Autodesk Inventor part; units mm, degrees
ref_plane "YZ Plane" through (0, 0, 0) normal (1, 0, 0) x (0, 1, 0)
ref_plane "XZ Plane" through (0, 0, 0) normal (0, 1, 0) x (-1, 0, 0)
ref_plane "XY Plane" through (0, 0, 0) normal (0, 0, 1) x (1, 0, 0)
sketch "Sketch1" plane through (0, 0, 0) normal (0, 0, 1) x (1, 0, 0)
  line L0 (0, 0) -> (101.4, 0)
  line L1 (101.4, 0) -> (101.4, 50)
  line L2 (101.4, 50) -> (0, 50)
  line L3 (0, 50) -> (0, 0)
  circle A0 centre (50.7, 25) radius 3.75
  line L4 (2.5, 36.45) -> (2.5, 13.55) construction
  line L5 (1.45, 36.45) -> (1.45, 13.55)
  line L6 (3.55, 13.55) -> (3.55, 36.45)
  arc A1 (3.55, 36.45) -> (1.45, 36.45) centre (2.5, 36.45) ccw
  arc A2 (1.45, 13.55) -> (3.55, 13.55) centre (2.5, 13.55) ccw
  line L7 (101.4, 50) -> (101.4, 0)
  line L8 (98.9, 36.45) -> (98.9, 13.55) construction
  line L9 (99.95, 36.45) -> (99.95, 13.55)
  line L10 (97.85, 13.55) -> (97.85, 36.45)
  arc A3 (99.95, 36.45) -> (97.85, 36.45) centre (98.9, 36.45) ccw
  arc A4 (97.85, 13.55) -> (99.95, 13.55) centre (98.9, 13.55) ccw
  point P0 (2.5, 25)
  point P1 (2.5, 12.5)
  point P2 (2.5, 37.5)
  point P3 (98.9, 25)
  point P4 (98.9, 12.5)
  point P5 (98.9, 37.5)
  point P6 (98.9, 25)
  dimension "d2" = 101.4
  dimension "d3" = 50
  dimension "d23" = 7.5
  dimension "d24" = 25
  dimension "d26" = 2.1
  dimension "d28" = 25
  dimension "d29" = 25
  dimension "d31" = 2.5
extrude "Extrusion1" add sketch "Sketch1" along normal mid plane 10
Read the model definition and answer for the solid it produces. Units are mm, in the model's axes. A direction names the side the tool comes from. Give positions to 0.01 mm unless a question says otherwise; leave off trailing zeros. Loops run counter-clockwise (first coordinate to the right, second up) from the corner with the lowest first, then second, coordinate; pieces in that order, holes last. Notation, with made-up numbers: (-34.75, -25) -> (10.25, -25) arc R17 cw to (10.25, -18) -> close; hole circle Ø3 at (10.25, -7.75). An arc over 180 degrees is marked (long way). Answer as CSV lines item,"result".
Item 1: Find section C-C on z = -0.5. Give the vertices of the cut face in (x, y), plus the area to 3 significant figures.
Returned:
outline,"(0, 0) -> (101.4, 0) -> (101.4, 50) -> (0, 50) -> close; hole (1.45, 13.55) arc R1.05 ccw to (3.55, 13.55) -> (3.55, 36.45) arc R1.05 ccw to (1.45, 36.45) -> close; hole circle Ø7.5 at (50.7, 25); hole (97.85, 13.55) arc R1.05 ccw to (99.95, 13.55) -> (99.95, 36.45) arc R1.05 ccw to (97.85, 36.45) -> close"
area,"4,920 mm²"
Item 2: Find section B-B on y = 15.5. Give the vertices of the cut face in (x, z).
Returned:
outline,"(0, -5) -> (1.45, -5) -> (1.45, 5) -> (0, 5) -> close; (3.55, -5) -> (97.85, -5) -> (97.85, 5) -> (3.55, 5) -> close; (99.95, -5) -> (101.4, -5) -> (101.4, 5) -> (99.95, 5) -> close"
Item 3: Determine the mould class of faces 3 (the face through (3.55, 25, 0)), 4 (the face through (1.45, 25, 0)), 5 (the face through (101.4, 25, 0)), 6 (the face through (50, 31, 5)) for opening direction X: +X half, -X half, draft (parallel to the pull), parting line (faces both ways), or undercut.
Returned:
face 3,"undercut"
face 4,"undercut"
face 5,"+X half"
face 6,"draft"
Item 4: Consider line 1 (X direction, y = 34, z = -1.5); line 2 (Y direction, x = 50.7, z = -1.5); line 3 (Y direction, x = 52.5, z = -2.5). Determine where each line is inside the solid, lowest interval first. Write a range as [from, to].
Returned:
line 1,"x = [0, 1.45], [3.55, 97.85], [99.95, 101.4]"
line 2,"y = [0, 21.25], [28.75, 50]"
line 3,"y = [0, 21.71], [28.29, 50]"
Item 5: Find section D-D on y = 27.5. Give the vertices of the cut face in (x, z), plus the area to 3 significant figures.
Returned:
outline,"(0, -5) -> (1.45, -5) -> (1.45, 5) -> (0, 5) -> close; (3.55, -5) -> (47.9, -5) -> (47.9, 5) -> (3.55, 5) -> close; (53.5, -5) -> (97.85, -5) -> (97.85, 5) -> (53.5, 5) -> close; (99.95, -5) -> (101.4, -5) -> (101.4, 5) -> (99.95, 5) -> close"
area,"916 mm²"
Item 6: For faces 1 (the face through (0, 25, 0)), 2 (the face through (98.9, 12.5, -0.1)), determine the directions among +Z, -Z, +X, -X, +Y, -Y from which every point of the face is accessible in a straight line to the end or side of a thin tool.
Returned:
face 1,"+Z, -Z, -X, +Y, -Y"
face 2,"+Z, -Z"
Item 7: Find section A-A on x = 50.7. Give the vertices of the cut face in (y, z).
Returned:
outline,"(0, -5) -> (21.25, -5) -> (21.25, 5) -> (0, 5) -> close; (28.75, -5) -> (50, -5) -> (50, 5) -> (28.75, 5) -> close"
